Part print with two shaded views. Sizes in mm from the minimum x, y, z corner. Round coordinates to 2 decimals unless told otherwise and drop trailing zeros. Loops run counter-clockwise (first coordinate to the right, second up) from the corner with the lowest first, then second, coordinate; pieces in that order, holes last.
(1) Cut at D-D on y = 2. List the corners of the cut face in (x, z).
(2) Probe probe 1 along X at (y, z) = (1.9, 40); probe 2 along Y at (x, z) = (52, 11); probe 3 along Z at (x, y) = (72.5, 14) (1 decimal). List the from-to ranges inside material, lowest first.
(3) Flat gauge pins, fed straight in: pin 1 (4 mm diameter, centred on x = 43, y = 14, fed in from +Z); pin 2 (4 mm diameter, centred on x = 8, y = 15, fed in from -Z); pin 3 (8 mm diameter, centred on x = 51, z = 22.5, fed in from +Y). Where does each tip first touch, or does it go through?
(4) Mould opens along Z. For the marked faces 1 and 2 say: +Z half, -Z half, draft (parallel to the pull), parting line (faces both ways), or undercut.
(5) Cut at B-B on x = 33. List the corners of the cut face in (y, z).
(6) Cut at C-C on z = 25. List the corners of the cut face in (x, y).
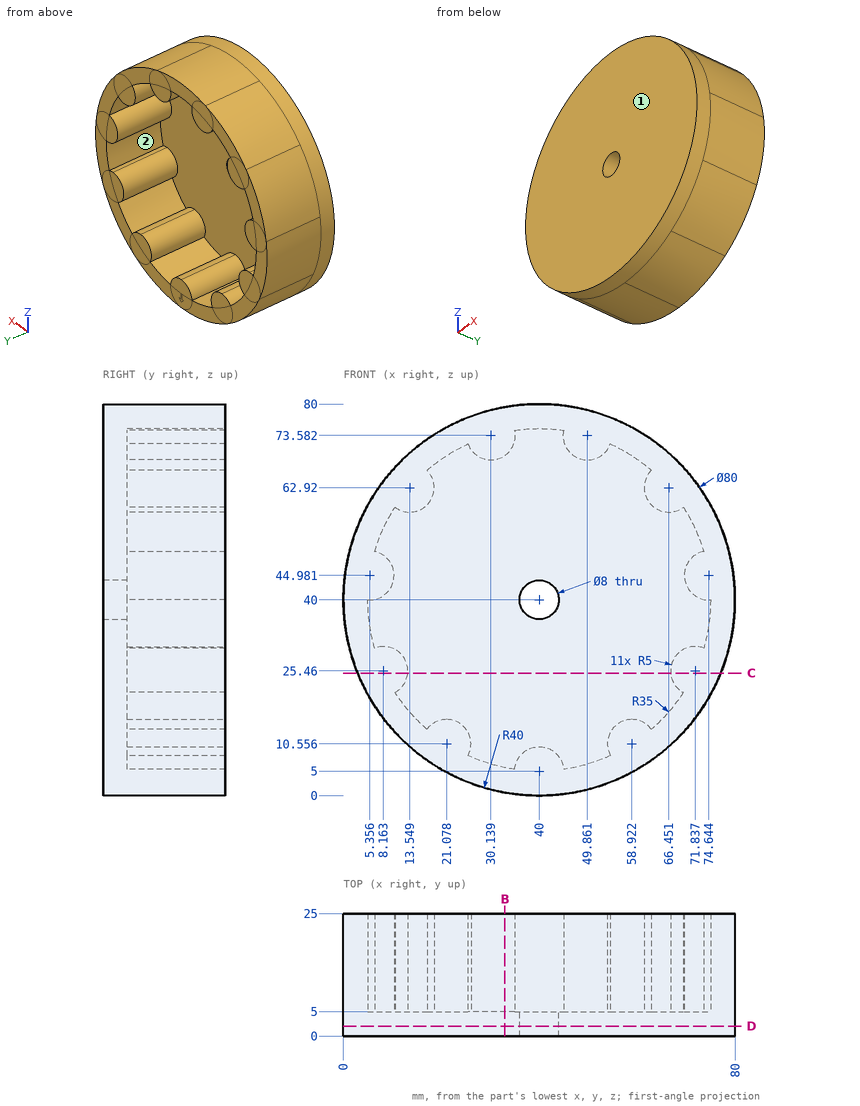
Final values:
1. outline: circle Ø80 at (40, 40); hole circle Ø8 at (40, 40)
2. probe 1: x = 0 to 36, 44 to 80
2. probe 2: y = 0 to 5
2. probe 3: z = 16.7 to 30.4, 40.5 to 49.5, 53 to 63.3
3. pin 1: stops at z = 79.99
3. pin 2: stops at z = 13.54
3. pin 3: stops at y = 5
4. face 1: draft
4. face 2: undercut
5. outline: (0, 0.62) - (25, 0.62) - (25, 5.71) - (5, 5.71) - (5, 69.48) - (25, 69.48) - (25, 79.38) - (0, 79.38) - close
6. outline: (2.92, 0) - (77.08, 0) - (77.08, 25) - (66.86, 25) - (66.86, 5) - (13.14, 5) - (13.14, 25) - (2.92, 25) - close
